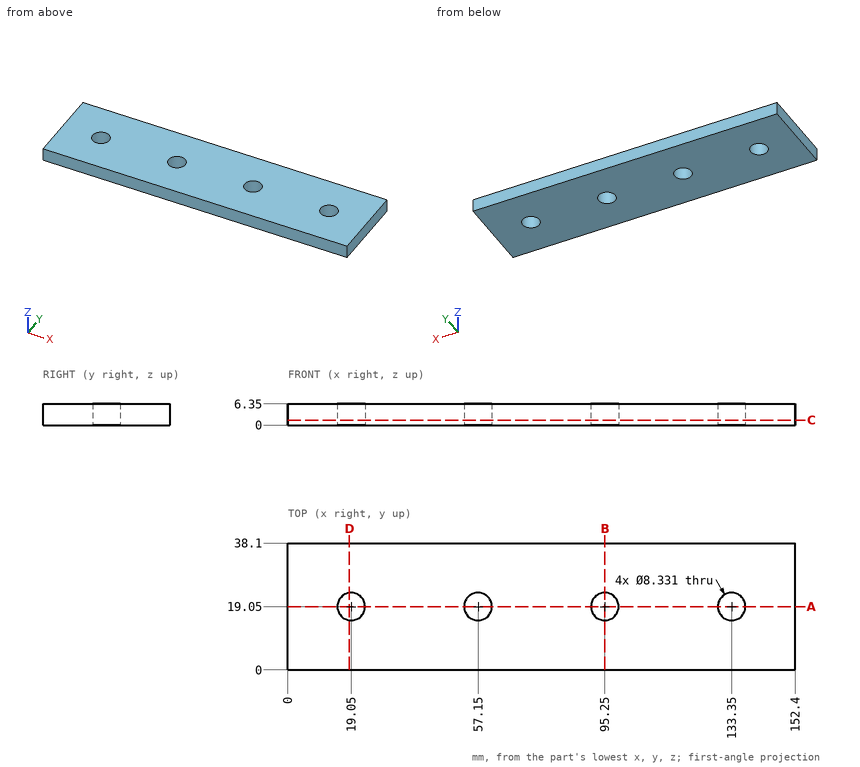
Source: three-view drawing plus pictorial views. Frame: mm from the lowest corner of the part. Round coordinates to 2 decimals unless told otherwise and drop trailing zeros. Write each loop counter-clockwise with the first axis right and the second up, starting at its lowest first coordinate (ties: lowest second). Pieces come first, ordered by that corner, then holes. Notation, with made-up numbers: M 31,56.25 L 82,56.25 A26 ccw 82,93.25 Z; hole C 43.5,4.5 d3. An arc over 180 degrees is marked long. Use CSV: the item, a comma, the result in double quotes. Start each with the question number.
Q1. Cut plane D-D on x = 18.5. Output: boundary loops of the cut face in (y, z).
Q2. Line query: line 1 (Y direction, x = 19.05, z = 2.5); line 2 (X direction, y = 18, z = 0.5); line 3 (X direction, y = 16.5, z = 6). Output: solid intervals per line, ascending. Write a range as from..to.
Q3. First-contact query: P1, Ø6.5, axis at x = 57.15, y = 19.05, coming from the +Z side. Flat tip, straight axial feed; report the tip coordinate or a pass-through.
Q4. Cut plane C-C on z = 1.5. Output: boundary loops of the cut face in (x, y).
Q5. Cut plane B-B on x = 95.25. Output: boundary loops of the cut face in (y, z).
Q6. Cut plane A-A on y = 19.05. Output: boundary loops of the cut face in (x, z).
Results found:
1,outline,"M 0,0 L 14.92,0 L 14.92,6.35 L 0,6.35 Z; M 23.18,0 L 38.1,0 L 38.1,6.35 L 23.18,6.35 Z"
2,line 1,"0..14.88, 23.22..38.1"
2,line 2,"0..15.02, 23.08..53.12, 61.18..91.22, 99.28..129.32, 137.38..152.4"
2,line 3,"0..15.76, 22.34..53.86, 60.44..91.96, 98.54..130.06, 136.64..152.4"
3,P1,"through"
4,outline,"M 0,0 L 152.4,0 L 152.4,38.1 L 0,38.1 Z; hole C 19.05,19.05 d8.33; hole C 57.15,19.05 d8.33; hole C 95.25,19.05 d8.33; hole C 133.35,19.05 d8.33"
5,outline,"M 0,0 L 14.88,0 L 14.88,6.35 L 0,6.35 Z; M 23.22,0 L 38.1,0 L 38.1,6.35 L 23.22,6.35 Z"
6,outline,"M 0,0 L 14.88,0 L 14.88,6.35 L 0,6.35 Z; M 23.22,0 L 52.98,0 L 52.98,6.35 L 23.22,6.35 Z; M 61.32,0 L 91.08,0 L 91.08,6.35 L 61.32,6.35 Z; M 99.42,0 L 129.18,0 L 129.18,6.35 L 99.42,6.35 Z; M 137.52,0 L 152.4,0 L 152.4,6.35 L 137.52,6.35 Z"
